The model under review builds one solid part; all positions refer to its coordinate system, in mm. A direction names the side the tool comes from. Round coordinates to 2 decimals unless told otherwise and drop trailing zeros. Loops run counter-clockwise (first coordinate to the right, second up) from the corner with the lowest first, then second, coordinate; pieces in that order, holes last. Notation, with made-up numbers: (5, 16) -> (28, 16) arc R25 ccw to (28, 55) -> close; hole circle Ø10 at (9, -30.5). An arc over 180 degrees is marked (long way). Write each question's results on one line, items separated by ' | '. Start each with the question number.
Item 1: We need section C-C (x = 1.25). Give the boundary of the cut face in (y, z) (3 decimals), and give its area (3 significant figures).
Item 2: Clearance check with flat-ended pins moving along their axes: pin 1 Ø8 at (x, y) = (-3.5, -2.5) entering from -Z; pin 2 Ø3.5 at (y, z) = (50.5, -20) entering from -X; pin 3 Ø1.5 at (x, z) = (-2, -9) entering from -Y; pin 4 Ø2.5 at (y, z) = (52.07, -17.653) entering from -X. State where each tip first meets the part, or that it passes through.
Item 3: We need section D-D (z = 0). Give the number of separate pieces and of enclosed holes in the cut face, and give its area (3 significant figures).
Item 4: For L1, parallel to Y at x = 1.5, z = -26; L2, parallel to Z at x = -6.5, y = 11; L3, parallel to X at y = -5.5, z = -0.5 (3 decimals), list the stretches that pass through material, from the lowest coordinate up. Write a range as from..to.
Item 5: Tool access review of faces 1 (the flat face through (-6, -49.658, -10)), 2 (the flat face through (-7, 6, -5.912)), 3 (the flat face through (2, 45.848, -19)), 4 (the flat face through (0, 50, -19)): name each direction out of +Z, -Z, +X, -X, +Y, -Y from which nothing blocks a thin tool from reaching the whole face with its end or side.
Item 6: Mouldability with a two-part tool opening along Z and no side actions: class faces 5 (the flat face through (-5, -45.848, -19)), 6 (the cylindrical face through (1.569, -22.964, 0.44)), 7 (the flat face through (2, -54, -8.5)) as pulls with the +Z half, pulls with the -Z half, needs draft (parallel to the pull), parting line crosses it, or undercut.
from build123d import *

# Parameters (mm, degrees)
BOSS_EXTRUDE1_DEPTH   = 3.175
BOSS_EXTRUDE2_DEPTH   = 12.60732
FILLET1_R             = 1.5875
FILLET2_R             = 3.175
CUT_EXTRUDE1_DEPTH    = 16
F_6_32_TAPPED_HOLE1_D = 2.7051
SKETCH10_R            = 2.667
CUT_EXTRUDE2_DEPTH    = 4.175
CHAMFER1_SIZE         = 0.254
FILLET3_R             = 1.5875
FILLET4_R             = 0.39624


with BuildPart() as part:
    # Sketch1 → Boss-Extrude1 (new body)
    with BuildSketch(Plane(origin=(0, 0, 0), x_dir=(0, 0, -1), z_dir=(1, 0, 0))):
        Polygon((27.813, 57.15), (27.813, 45.847999998), (7.5, 45.847999998), (7.5, -45.847999998), (27.813, -45.847999998), (27.813, -57.15), (8.5, -57.15), (8.5, -49.657999998), (-7.5, -49.657999998), (-7.5, 57.15), align=None)
    extrude(amount=BOSS_EXTRUDE1_DEPTH)

    # Sketch2 → Boss-Extrude2 (add)
    with BuildSketch(Plane.ZY):
        Polygon((7.5, -49.657999998), (7.5, -45.847999998), (-5.9125, -45.847999998), (-5.9125, 57.15), (-7.5, 57.15), (-7.5, -45.847999998), (-27.813, -45.847999998), (-27.813, -49.657999998), align=None)
    extrude(amount=BOSS_EXTRUDE2_DEPTH)

    # Sketch4 → #10 Clearance Hole1 (revolve, cut)
    with BuildSketch(Plane(origin=(-5.10794, -49.657999998, 0), x_dir=(0, 0, -1), z_dir=(1, 0, 0))):
        Polygon((0, 0), (0, 3.81), (3.1242, 3.81), (2.4892, 3.175), (2.4892, 0.635), (3.1242, 0), align=None)
    revolve(axis=Axis((-5.10794, -56.007999998, 0), (0, 1, 0)), mode=Mode.SUBTRACT)

    # Fillet1
    fillet1_edges = [part.edges().sort_by_distance(p)[0] for p in [
        (-6.30366, -45.847999998, -5.9125),
    ]]
    fillet(fillet1_edges, radius=FILLET1_R)

    # Fillet2
    fillet2_edges = [part.edges().sort_by_distance(p)[0] for p in [
        (-4.71616, -45.847999998, -7.5),
        (1.5875, 45.847999998, -7.5),
    ]]
    fillet(fillet2_edges, radius=FILLET2_R)

    # Sketch6 → Cut-Extrude1 (cut, through all)
    with BuildSketch(Plane(origin=(0, 0, -7.5), x_dir=(-1, 0, 0), z_dir=(0, 0, -1))):
        Polygon((2.447319972, 57.15), (12.607319972, 57.15), (12.607319972, 46.99), align=None)
    extrude(amount=-CUT_EXTRUDE1_DEPTH, mode=Mode.SUBTRACT)

    # #6-32 Tapped Hole1 (through all)
    with Locations(Plane(origin=(3.175, 0, 0), x_dir=(0, 0, -1), z_dir=(1, 0, 0))):
        with Locations((17.653, 52.07)):
            f_6_32_tapped_hole1 = Hole(F_6_32_TAPPED_HOLE1_D / 2)

    # Sketch10 → Cut-Extrude2 (cut, through all)
    with BuildSketch(Plane.ZY):
        with Locations((0.7874, 20.32)):
            Circle(SKETCH10_R)
    cut_extrude2 = extrude(amount=-CUT_EXTRUDE2_DEPTH, mode=Mode.SUBTRACT)

    # Mirror2: Cut-Extrude2 across plane
    add(cut_extrude2.mirror(Plane.ZX), mode=Mode.SUBTRACT)

    # Chamfer1
    chamfer1_edges = [part.edges().sort_by_distance(p)[0] for p in [
        (3.175, 20.32, -1.8796),
        (0, 20.32, -1.8796),
        (3.175, -20.32, -1.8796),
        (0, -20.32, -1.8796),
    ]]
    chamfer(chamfer1_edges, length=CHAMFER1_SIZE)

    # Fillet3
    fillet3_edges = [part.edges().sort_by_distance(p)[0] for p in [
        (0, 6.444750001, -5.9125),
        (0, -45.383032013, -5.447532015),
        (0, -49.657999998, -18.1565),
        (0, 49.911499999, -7.5),
        (0, -45.847999998, 1.5875),
    ]]
    fillet(fillet3_edges, radius=FILLET3_R)

    # Mirror1: #6-32 Tapped Hole1 across plane
    add(f_6_32_tapped_hole1.mirror(Plane.ZX), mode=Mode.SUBTRACT)

    # Fillet4
    fillet4_edges = [part.edges().sort_by_distance(p)[0] for p in [
        (0.79375, -49.657999998, -8.5),
    ]]
    fillet(fillet4_edges, radius=FILLET4_R)


solid = part.part
Here are the results:
1) outline: (-57.15, -27.813) -> (-45.848, -27.813) -> (-45.848, -10.675) arc R3.175 cw to (-42.673, -7.5) -> (42.673, -7.5) arc R3.175 cw to (45.848, -10.675) -> (45.848, -27.813) -> (57.15, -27.813) -> (57.15, 7.5) -> (-49.658, 7.5) -> (-49.658, -8.104) arc R0.396 cw to (-50.054, -8.5) -> (-57.15, -8.5) -> close; hole circle Ø2.705 at (-52.07, -17.653); hole circle Ø5.334 at (-20.32, 0.787); hole circle Ø5.334 at (20.32, 0.787); hole circle Ø2.705 at (52.07, -17.653) | area: 2,000 mm2
2) pin 1: stops at z = -7.5 | pin 2: stops at x = 0 | pin 3: stops at y = -49.69 | pin 4: passes through
3) separate pieces: 4 | enclosed holes: 0 | area: 335 mm2
4) L1: y = -57.15..-45.85, 45.85..57.15 | L2: z = -7.5..-5.91 | L3: x = 0..3.175
5) face 1: +Z, -X, -Y | face 2: +Z, -X, +Y | face 3: -Z, +X, -X | face 4: -Z, -X, +Y
6) face 5: needs draft | face 6: undercut | face 7: pulls with the +Z half
